Build history of the part. All positions in model axes, mm. A direction names the side the tool comes from. Round coordinates to 2 decimals unless told otherwise and drop trailing zeros. Write each loop counter-clockwise with the first axis right and the second up, starting at its lowest first coordinate (ties: lowest second). Pieces come first, ordered by that corner, then holes. Notation, with made-up numbers: (46.25, 42) -> (94.25, 42) arc R17 ccw to (94.25, 48) -> close; hole circle Ø10 at (-40, -37.75). An arc over 180 degrees is marked (long way). One line per question, with ' | ' between items.
from build123d import *

# Parameters (mm, degrees)
SKETCH1_R               = 21
BOSS_EXTRUDE1_DEPTH     = 100
SKETCH3_R               = 3.5
BOSS_EXTRUDE3_DEPTH     = 26
SKETCH4_R               = 7
BOSS_EXTRUDE4_DEPTH     = 7
SKETCH5_W               = 43
SKETCH5_H               = 43
BOSS_EXTRUDE5_DEPTH     = 7
CUT_EXTRUDE1_DEPTH      = 105.52033295
CUT_EXTRUDE1_DEPTH_BACK = 105.52033295


with BuildPart() as part:
    # Sketch1 → Boss-Extrude1 (new body)
    with BuildSketch(Plane(origin=(0, 0, 0), x_dir=(1, 0, 0), z_dir=(0, 1, 0))):
        with Locations(Location((0, 0, 0), (0, 0, 270))):
            Circle(SKETCH1_R)
    extrude(amount=BOSS_EXTRUDE1_DEPTH)

    # Sketch3 → Boss-Extrude3 (add)
    with BuildSketch(Plane.XZ):
        with Locations(Location((0, 0, 0), (0, 0, 90))):
            Circle(SKETCH3_R)
    extrude(amount=BOSS_EXTRUDE3_DEPTH)

    # Sketch4 → Boss-Extrude4 (add)
    with BuildSketch(Plane.XZ):
        with Locations(Location((0, 0, 0), (0, 0, 90))):
            Circle(SKETCH4_R)
    extrude(amount=BOSS_EXTRUDE4_DEPTH)

    # Sketch5 → Boss-Extrude5 (add)
    with BuildSketch(Plane.XZ):
        Rectangle(SKETCH5_W, SKETCH5_H)
    extrude(amount=-BOSS_EXTRUDE5_DEPTH)

    # Sketch6 → Cut-Extrude1 (cut, two sides: drawn at the far end of the back side and taken through both)
    with BuildSketch(Plane.XZ.offset(-CUT_EXTRUDE1_DEPTH_BACK)):
        with BuildLine():
            ThreePointArc((-16, 18), (-19.414213562, 19.414213562), (-18, 16))
            Line((-18, 16), (-18, 18))
            Line((-18, 18), (-16, 18))
        make_face()
        with BuildLine():
            Line((-18, 18), (-18, 16))
            ThreePointArc((-18, 16), (-16.585786438, 16.585786438), (-16, 18))
            Line((-16, 18), (-18, 18))
        make_face()
        with BuildLine():
            Line((-18, -16), (-18, -18))
            Line((-18, -18), (-16, -18))
            ThreePointArc((-16, -18), (-16.585786438, -16.585786438), (-18, -16))
        make_face()
        with BuildLine():
            Line((-16, -18), (-18, -18))
            Line((-18, -18), (-18, -16))
            ThreePointArc((-18, -16), (-19.414213562, -19.414213562), (-16, -18))
        make_face()
        with BuildLine():
            ThreePointArc((18, -16), (16.585786438, -16.585786438), (16, -18))
            Line((16, -18), (18, -18))
            Line((18, -18), (18, -16))
        make_face()
        with BuildLine():
            Line((18, -18), (16, -18))
            ThreePointArc((16, -18), (18, -20), (20, -18))
            ThreePointArc((20, -18), (19.414213562, -16.585786438), (18, -16))
            Line((18, -16), (18, -18))
        make_face()
        with BuildLine():
            ThreePointArc((16, 18), (16.585786438, 16.585786438), (18, 16))
            Line((18, 16), (18, 18))
            Line((18, 18), (16, 18))
        make_face()
        with BuildLine():
            Line((18, 18), (18, 16))
            ThreePointArc((18, 16), (19.414213562, 16.585786438), (20, 18))
            ThreePointArc((20, 18), (18, 20), (16, 18))
            Line((16, 18), (18, 18))
        make_face()
    extrude(amount=CUT_EXTRUDE1_DEPTH + CUT_EXTRUDE1_DEPTH_BACK, mode=Mode.SUBTRACT)


solid = part.part
(1) Slice it at D-D (x = -10). Write the cut outline in (y, z).
Calculated:
outline: (0, -21.5) -> (7, -21.5) -> (7, -18.47) -> (100, -18.47) -> (100, 18.47) -> (7, 18.47) -> (7, 21.5) -> (0, 21.5) -> close
(2) Slice it at A-A (z = 0). Write the cut outline in (x, y).
Calculated:
outline: (-21.5, 0) -> (-7, 0) -> (-7, -7) -> (-3.5, -7) -> (-3.5, -26) -> (3.5, -26) -> (3.5, -7) -> (7, -7) -> (7, 0) -> (21.5, 0) -> (21.5, 7) -> (21, 7) -> (21, 100) -> (-21, 100) -> (-21, 7) -> (-21.5, 7) -> close
(3) Drop flat-ended pins along their axis: pin 1 (12 mm diameter, centred on x = 11.5, y = 45.5, fed in from +Z); pin 2 (4.5 mm diameter, centred on x = -18, z = 18, fed in from +Y); pin 3 (8 mm diameter, centred on y = 37, z = -15, fed in from -X). Give the stop position or say it passes through.
Calculated:
pin 1: z = 20.27 | pin 2: y = 7 | pin 3: x = -17.89
(4) Slice it at B-B (x = 0). Write the cut outline in (y, z), then the cut area to 3 significant figures.
Calculated:
outline: (-26, -3.5) -> (-7, -3.5) -> (-7, -7) -> (0, -7) -> (0, -21.5) -> (7, -21.5) -> (7, -21) -> (100, -21) -> (100, 21) -> (7, 21) -> (7, 21.5) -> (0, 21.5) -> (0, 7) -> (-7, 7) -> (-7, 3.5) -> (-26, 3.5) -> close | area: 4,440 mm2
(5) Slice it at C-C (y = 32). Write the cut outline in (x, z), then the cut area to 3 significant figures.
Calculated:
outline: circle Ø42 at (0, 0) | area: 1,390 mm2
(6) 3-axis set-ups, long thin cutter, end or side, ignore diameter. For faces 1 (the flat face through (-21.5, 3, 0)), 2 (the cylindrical face through (6.31, 52.85, 20.03)), 3 (the flat face through (3, -7, 3)): which of +Z, -Z, +X, -X, +Y, -Y reach the whole face in a straight line?
Calculated:
face 1: +Z, -Z, -X, +Y, -Y | face 2: +Y | face 3: -Y
(7) Wall check: line 1 (X direction, y = 3.5, z = 18); line 2 (Y direction, x = 17, z = -2.5). Give the ranges that are in metal, low to high. Write a range as from..to.
Calculated:
line 1: -21.5..-20, -16..16, 20..21.5 | line 2: 0..100
